```python
from build123d import *

# Parameters (mm, degrees)
SKETCH1_W                       = 105
SKETCH1_H                       = 190
BASE_FLANGE1_DEPTH              = 3
EDGE_FLANGE1_STRIP_W            = 13.4732
EDGE_FLANGE1_STRIP_H            = 3
EDGE_FLANGE1_STRIP_CUT_DEPTH    = 190
EDGE_FLANGE1_STRIP_2_W          = 13.4732
EDGE_FLANGE1_STRIP_2_H          = 3
EDGE_FLANGE1_STRIP_CUT_2_DEPTH  = 190
EDGE_FLANGE1_DEPTH              = 190
EDGE_FLANGE1_BEND_DEPTH         = 190
SKETCH33_R                      = 4.25
CUT_EXTRUDE1_DEPTH              = 10
EDGE_FLANGE8_STRIP_W            = 13.4732
EDGE_FLANGE8_STRIP_H            = 3
EDGE_FLANGE8_STRIP_CUT_DEPTH    = 190
EDGE_FLANGE8_STRIP_2_W          = 13.4732
EDGE_FLANGE8_STRIP_2_H          = 3
EDGE_FLANGE8_STRIP_CUT_2_DEPTH  = 190
EDGE_FLANGE8_DEPTH              = 190
EDGE_FLANGE8_BEND_DEPTH         = 190
EDGE_FLANGE9_STRIP_W            = 13.4732
EDGE_FLANGE9_STRIP_H            = 3
EDGE_FLANGE9_STRIP_CUT_DEPTH    = 190
EDGE_FLANGE9_STRIP_2_W          = 13.4732
EDGE_FLANGE9_STRIP_2_H          = 3
EDGE_FLANGE9_STRIP_CUT_2_DEPTH  = 190
EDGE_FLANGE9_DEPTH              = 190
EDGE_FLANGE9_BEND_DEPTH         = 190
EDGE_FLANGE10_STRIP_W           = 13.4732
EDGE_FLANGE10_STRIP_H           = 3
EDGE_FLANGE10_STRIP_CUT_DEPTH   = 190
EDGE_FLANGE10_STRIP_2_W         = 13.4732
EDGE_FLANGE10_STRIP_2_H         = 3
EDGE_FLANGE10_STRIP_CUT_2_DEPTH = 190
EDGE_FLANGE10_DEPTH             = 190
EDGE_FLANGE10_BEND_DEPTH        = 190
SKETCH72_R                      = 4.25
CUT_EXTRUDE4_DEPTH              = 10
CUT_EXTRUDE5_START              = -10
SKETCH77_R                      = 4.25
CUT_EXTRUDE5_DEPTH              = 10
SKETCH78_R                      = 4.25
CUT_EXTRUDE8_DEPTH              = 10


# Sheet-metal steps are written as plain solids
with BuildPart() as part:
    # Sketch1 → Base-Flange1 (new body)
    with BuildSketch(Plane(origin=(0, 0, 0), x_dir=(1, 0, 0), z_dir=(0, 1, 0))):
        Rectangle(SKETCH1_W, SKETCH1_H)
    extrude(amount=-BASE_FLANGE1_DEPTH)

    # Edge-Flange1 strip (across the edge) → Edge-Flange1 strip cut (cut)
    with BuildSketch(Plane(origin=(52.5, 0, 95), x_dir=(-1, 0, 0), z_dir=(0, 0, -1))):
        with Locations((-3, -1.5)):
            Rectangle(EDGE_FLANGE1_STRIP_W, EDGE_FLANGE1_STRIP_H)
    extrude(amount=EDGE_FLANGE1_STRIP_CUT_DEPTH, mode=Mode.SUBTRACT)

    # Edge-Flange1 strip 2 (across the edge) → Edge-Flange1 strip cut 2 (cut)
    with BuildSketch(Plane(origin=(-52.5, 0, -95), x_dir=(1, 0, 0), z_dir=(0, 0, 1))):
        with Locations((-3, -1.5)):
            Rectangle(EDGE_FLANGE1_STRIP_2_W, EDGE_FLANGE1_STRIP_2_H)
    extrude(amount=EDGE_FLANGE1_STRIP_CUT_2_DEPTH, mode=Mode.SUBTRACT)

    # Edge-Flange1 section (across the edge) → Edge-Flange1 (add)
    with BuildSketch(Plane(origin=(52.5, 0, 95), x_dir=(-1, 0, 0), z_dir=(0, 0, -1))):
        with BuildLine():
            Line((0, 0.7366), (0, 7))
            Line((0, 7), (3, 7))
            Line((3, 7), (3, 0.7366))
            ThreePointArc((3, 0.7366), (3.215745145, 0.215745145), (3.7366, 0))
            Line((3.7366, 0), (3.7366, -3))
            ThreePointArc((3.7366, -3), (1.094424801, -1.905575199), (0, 0.7366))
        make_face()
    extrude(amount=EDGE_FLANGE1_DEPTH)

    # Edge-Flange1 section 2 (across the edge) → Edge-Flange1 bend (add)
    with BuildSketch(Plane(origin=(-52.5, 0, -95), x_dir=(1, 0, 0), z_dir=(0, 0, 1))):
        with BuildLine():
            Line((0, 0.7366), (0, 7))
            Line((0, 7), (3, 7))
            Line((3, 7), (3, 0.7366))
            ThreePointArc((3, 0.7366), (3.215745145, 0.215745145), (3.7366, 0))
            Line((3.7366, 0), (3.7366, -3))
            ThreePointArc((3.7366, -3), (1.094424801, -1.905575199), (0, 0.7366))
        make_face()
    extrude(amount=EDGE_FLANGE1_BEND_DEPTH)

    # Sketch33 → Cut-Extrude1 (cut)
    with BuildSketch(Plane(origin=(0, 0, 0), x_dir=(1, 0, 0), z_dir=(0, 1, 0))):
        with Locations(Location((24.3834, -65, 0), (0, 0, 270))):
            Circle(SKETCH33_R)
        with Locations(Location((24.3834, 65, 0), (0, 0, 270))):
            Circle(SKETCH33_R)
        with Locations(Location((-24.3834, 65, 0), (0, 0, 270))):
            Circle(SKETCH33_R)
        with Locations(Location((-24.3834, -65, 0), (0, 0, 270))):
            Circle(SKETCH33_R)
    extrude(amount=-CUT_EXTRUDE1_DEPTH, mode=Mode.SUBTRACT)

    # Edge-Flange8 strip (across the edge) → Edge-Flange8 strip cut (cut)
    with BuildSketch(Plane(origin=(-52.5, 7, 95), x_dir=(0, -1, 0), z_dir=(0, 0, -1))):
        with Locations((-6, -1.5)):
            Rectangle(EDGE_FLANGE8_STRIP_W, EDGE_FLANGE8_STRIP_H)
    extrude(amount=EDGE_FLANGE8_STRIP_CUT_DEPTH, mode=Mode.SUBTRACT)

    # Edge-Flange8 strip 2 (across the edge) → Edge-Flange8 strip cut 2 (cut)
    with BuildSketch(Plane(origin=(52.5, 7, -95), x_dir=(0, -1, 0), z_dir=(0, 0, 1))):
        with Locations((-6, -1.5)):
            Rectangle(EDGE_FLANGE8_STRIP_2_W, EDGE_FLANGE8_STRIP_2_H)
    extrude(amount=EDGE_FLANGE8_STRIP_CUT_2_DEPTH, mode=Mode.SUBTRACT)

    # Edge-Flange8 section (across the edge) → Edge-Flange8 (add)
    with BuildSketch(Plane(origin=(-52.5, 7, 95), x_dir=(0, -1, 0), z_dir=(0, 0, -1))):
        with BuildLine():
            Line((-3, 0.7366), (-3, 15))
            Line((-3, 15), (0, 15))
            Line((0, 15), (0, 0.7366))
            ThreePointArc((0, 0.7366), (0.215745145, 0.215745145), (0.7366, 0))
            Line((0.7366, 0), (0.7366, -3))
            ThreePointArc((0.7366, -3), (-1.905575199, -1.905575199), (-3, 0.7366))
        make_face()
    extrude(amount=EDGE_FLANGE8_DEPTH)

    # Edge-Flange8 section 2 (across the edge) → Edge-Flange8 bend (add)
    with BuildSketch(Plane(origin=(52.5, 7, -95), x_dir=(0, -1, 0), z_dir=(0, 0, 1))):
        with BuildLine():
            Line((-3, 0.7366), (-3, 15))
            Line((-3, 15), (0, 15))
            Line((0, 15), (0, 0.7366))
            ThreePointArc((0, 0.7366), (0.215745145, 0.215745145), (0.7366, 0))
            Line((0.7366, 0), (0.7366, -3))
            ThreePointArc((0.7366, -3), (-1.905575199, -1.905575199), (-3, 0.7366))
        make_face()
    extrude(amount=EDGE_FLANGE8_BEND_DEPTH)

    # Edge-Flange9 strip (across the edge) → Edge-Flange9 strip cut (cut)
    with BuildSketch(Plane(origin=(-67.5, 10, -95), x_dir=(1, 0, 0), z_dir=(0, 0, 1))):
        with Locations((-6, -1.5)):
            Rectangle(EDGE_FLANGE9_STRIP_W, EDGE_FLANGE9_STRIP_H)
    extrude(amount=EDGE_FLANGE9_STRIP_CUT_DEPTH, mode=Mode.SUBTRACT)

    # Edge-Flange9 strip 2 (across the edge) → Edge-Flange9 strip cut 2 (cut)
    with BuildSketch(Plane(origin=(67.5, 10, 95), x_dir=(-1, 0, 0), z_dir=(0, 0, -1))):
        with Locations((-6, -1.5)):
            Rectangle(EDGE_FLANGE9_STRIP_2_W, EDGE_FLANGE9_STRIP_2_H)
    extrude(amount=EDGE_FLANGE9_STRIP_CUT_2_DEPTH, mode=Mode.SUBTRACT)

    # Edge-Flange9 section (across the edge) → Edge-Flange9 (add)
    with BuildSketch(Plane(origin=(-67.5, 10, -95), x_dir=(1, 0, 0), z_dir=(0, 0, 1))):
        with BuildLine():
            Line((-3, 0.7366), (-3, 15))
            Line((-3, 15), (0, 15))
            Line((0, 15), (0, 0.7366))
            ThreePointArc((0, 0.7366), (0.215745145, 0.215745145), (0.7366, 0))
            Line((0.7366, 0), (0.7366, -3))
            ThreePointArc((0.7366, -3), (-1.905575199, -1.905575199), (-3, 0.7366))
        make_face()
    extrude(amount=EDGE_FLANGE9_DEPTH)

    # Edge-Flange9 section 2 (across the edge) → Edge-Flange9 bend (add)
    with BuildSketch(Plane(origin=(67.5, 10, 95), x_dir=(-1, 0, 0), z_dir=(0, 0, -1))):
        with BuildLine():
            Line((-3, 0.7366), (-3, 15))
            Line((-3, 15), (0, 15))
            Line((0, 15), (0, 0.7366))
            ThreePointArc((0, 0.7366), (0.215745145, 0.215745145), (0.7366, 0))
            Line((0.7366, 0), (0.7366, -3))
            ThreePointArc((0.7366, -3), (-1.905575199, -1.905575199), (-3, 0.7366))
        make_face()
    extrude(amount=EDGE_FLANGE9_BEND_DEPTH)

    # Edge-Flange10 strip (across the edge) → Edge-Flange10 strip cut (cut)
    with BuildSketch(Plane(origin=(-67.5, 25, -95), x_dir=(0, -1, 0), z_dir=(0, 0, 1))):
        with Locations((-6, -1.5)):
            Rectangle(EDGE_FLANGE10_STRIP_W, EDGE_FLANGE10_STRIP_H)
    extrude(amount=EDGE_FLANGE10_STRIP_CUT_DEPTH, mode=Mode.SUBTRACT)

    # Edge-Flange10 strip 2 (across the edge) → Edge-Flange10 strip cut 2 (cut)
    with BuildSketch(Plane(origin=(67.5, 25, 95), x_dir=(0, -1, 0), z_dir=(0, 0, -1))):
        with Locations((-6, -1.5)):
            Rectangle(EDGE_FLANGE10_STRIP_2_W, EDGE_FLANGE10_STRIP_2_H)
    extrude(amount=EDGE_FLANGE10_STRIP_CUT_2_DEPTH, mode=Mode.SUBTRACT)

    # Edge-Flange10 section (across the edge) → Edge-Flange10 (add)
    with BuildSketch(Plane(origin=(-67.5, 25, -95), x_dir=(0, -1, 0), z_dir=(0, 0, 1))):
        with BuildLine():
            Line((-3, 0.7366), (-3, 15))
            Line((-3, 15), (0, 15))
            Line((0, 15), (0, 0.7366))
            ThreePointArc((0, 0.7366), (0.215745145, 0.215745145), (0.7366, 0))
            Line((0.7366, 0), (0.7366, -3))
            ThreePointArc((0.7366, -3), (-1.905575199, -1.905575199), (-3, 0.7366))
        make_face()
    extrude(amount=EDGE_FLANGE10_DEPTH)

    # Edge-Flange10 section 2 (across the edge) → Edge-Flange10 bend (add)
    with BuildSketch(Plane(origin=(67.5, 25, 95), x_dir=(0, -1, 0), z_dir=(0, 0, -1))):
        with BuildLine():
            Line((-3, 0.7366), (-3, 15))
            Line((-3, 15), (0, 15))
            Line((0, 15), (0, 0.7366))
            ThreePointArc((0, 0.7366), (0.215745145, 0.215745145), (0.7366, 0))
            Line((0.7366, 0), (0.7366, -3))
            ThreePointArc((0.7366, -3), (-1.905575199, -1.905575199), (-3, 0.7366))
        make_face()
    extrude(amount=EDGE_FLANGE10_BEND_DEPTH)

    # Sketch72 → Cut-Extrude4 (cut)
    with BuildSketch(Plane(origin=(70.5, 0, 0), x_dir=(0, 0, -1), z_dir=(1, 0, 0))):
        with Locations(Location((0, 17.5, 0), (0, 0, 90))):
            Circle(SKETCH72_R)
    extrude(amount=-CUT_EXTRUDE4_DEPTH, mode=Mode.SUBTRACT)

    # Sketch77 → Cut-Extrude5 (cut)
    with BuildSketch(Plane.ZY.offset(70.5).offset(CUT_EXTRUDE5_START)):
        with Locations(Location((0, 17.5, 0), (0, 0, 90))):
            Circle(SKETCH77_R)
    extrude(amount=CUT_EXTRUDE5_DEPTH, mode=Mode.SUBTRACT)

    # Sketch78 → Cut-Extrude8 (cut)
    with BuildSketch(Plane(origin=(0, 0, 0), x_dir=(1, 0, 0), z_dir=(0, 1, 0))):
        with Locations(Location((0, -83.75, 0), (0, 0, 270))):
            Circle(SKETCH78_R)
    extrude(amount=-CUT_EXTRUDE8_DEPTH, mode=Mode.SUBTRACT)


solid = part.part
```
Geometry check sheet. Reference: the model listing, model coordinates, mm. A direction names the side the tool comes from. Give positions to 0.01 mm unless a question says otherwise; leave off trailing zeros. Write each loop counter-clockwise with the first axis right and the second up, starting at its lowest first coordinate (ties: lowest second). Pieces come first, ordered by that corner, then holes. Notation, with made-up numbers: (-15.5, 70.25) -> (9.5, 70.25) arc R29 ccw to (9.5, 104.25) -> close; hole circle Ø7 at (21.5, 49.5). An arc over 180 degrees is marked (long way). Use one line per item in the form item = value.
Item 1: Mould release check, pull along X, two halves, no side actions. Record for faces 1 (the cylindrical face through (25.66, -1.479, 69.054)), 2 (the cylindrical face through (69.43, 26.88, 1.33)), 3 (the flat face through (-70.5, 13, -1)), 4 (the flat face through (-60, 28, -1)): released by +X, released by -X, zero draft, split by the parting line, or undercut.
Results list:
face_1 = undercut
face_2 = released by +X
face_3 = released by -X
face_4 = zero draft
Item 2: Sectioned sample at B-B on x = -2. Enter the section's corners in (y, z), plus the area to 4 significant figures.
Results list:
outline = (-3, -95) -> (0, -95) -> (0, 80) -> (-3, 80) -> close; (-3, 87.5) -> (0, 87.5) -> (0, 95) -> (-3, 95) -> close
area = 547.5 mm2
Item 3: Sectioned sample at C-C on y = 4. Enter the section's corners in (x, z), plus the area to 3 significant figures.
Results list:
outline = (-52.5, -95) -> (-49.5, -95) -> (-49.5, 95) -> (-52.5, 95) -> close; (49.5, -95) -> (52.5, -95) -> (52.5, 95) -> (49.5, 95) -> close
area = 1,140 mm2
Item 4: Sectioned sample at D-D on z = 65. Count the separate pieces of the cut face and the enclosed holes in it, plus the area to 3 significant figures.
Results list:
separate_pieces = 3
enclosed_holes = 0
area = 607 mm2
Item 5: Access from +Z, -Z, +X, -X, +Y, -Y to the whole of each face (thin tool, end or side, straight path). Record for faces 5 (the flat face through (49.5, 4, 1)), 6 (the flat face through (4.9, -0.2, 95)), 7 (the flat face through (-60, 7, 1)), 8 (the flat face through (67.5, 22, 1)).
Results list:
face_5 = +Z, -Z, +Y
face_6 = +Z, +X, -X, +Y, -Y
face_7 = +Z, -Z, -X, -Y
face_8 = +Z, -Z
Item 6: Depth check by flat-ended pin: pin 1 Ø1.5 at (y, z) = (26.5, -4) entering from +X; pin 2 Ø7.5 at (x, z) = (24.38, -65) entering from -Y; pin 3 Ø3 at (y, z) = (4.5, -30.5) entering from -X; pin 4 Ø4 at (x, z) = (-3.5, 41.5) entering from +Y. Enter the tip coordinate at first touch or a pass-through.
Results list:
pin_1 = 70.19
pin_2 = through
pin_3 = -52.5
pin_4 = 0
Item 7: Scan lines: line 1 (X direction, y = 18.5, z = -38.5); line 2 (X direction, y = -2.35, z = 65); line 3 (Z direction, x = -68.4, y = 17.5). Record each from-to range of solid material in increasing order.
Results list:
line_1 = -70.5 to -67.5, 67.5 to 70.5
line_2 = -50.87 to -28.63, -20.13 to 20.13, 28.63 to 50.87
line_3 = -95 to -4.25, 4.25 to 95
Item 8: Sectioned sample at A-A on y = 17.5. Enter the section's corners in (x, z).
Results list:
outline = (-70.5, -95) -> (-67.5, -95) -> (-67.5, -4.25) -> (-70.5, -4.25) -> close; (-70.5, 4.25) -> (-67.5, 4.25) -> (-67.5, 95) -> (-70.5, 95) -> close; (67.5, -95) -> (70.5, -95) -> (70.5, -4.25) -> (67.5, -4.25) -> close; (67.5, 4.25) -> (70.5, 4.25) -> (70.5, 95) -> (67.5, 95) -> close
